from build123d import *

# Parameters (mm, degrees)
SKETCH1_R           = 2.5
SKETCH1_R_2         = 0.5
BOSS_EXTRUDE2_DEPTH = 4.572


with BuildPart() as part:
    # Sketch1 → Boss-Extrude2 (new body)
    with BuildSketch(Plane.XY):
        with BuildLine():
            Line((4.800174543, 7.530126516), (4.800174543, 44.360126516))
            ThreePointArc((4.800174543, 44.360126516), (4.056225767, 46.15617774), (2.260174543, 46.900126516))
            Line((2.260174543, 46.900126516), (-2.819825457, 46.900126516))
            ThreePointArc((-2.819825457, 46.900126516), (-4.615876681, 46.15617774), (-5.359825457, 44.360126516))
            Line((-5.359825457, 44.360126516), (-5.359825457, -5.169873484))
            Line((-5.359825457, -5.169873484), (-5.359825457, -47.079873484))
            ThreePointArc((-5.359825457, -47.079873484), (28.060725855, -35.300861478), (46.710174543, -5.169873484))
            Line((46.710174543, -5.169873484), (46.710174543, -2.629873484))
            Line((46.710174543, -2.629873484), (46.710174543, 2.450126516))
            ThreePointArc((46.710174543, 2.450126516), (45.966225767, 4.24617774), (44.170174543, 4.990126516))
            Line((44.170174543, 4.990126516), (7.340174543, 4.990126516))
            ThreePointArc((7.340174543, 4.990126516), (5.544123319, 5.734075291), (4.800174543, 7.530126516))
        make_face()
        Circle(SKETCH1_R, mode=Mode.SUBTRACT)
        with Locations((0, 11.43)):
            Circle(SKETCH1_R_2, mode=Mode.SUBTRACT)
        with Locations((11.43, 0)):
            Circle(SKETCH1_R_2, mode=Mode.SUBTRACT)
        with Locations((0, 13.97)):
            Circle(SKETCH1_R_2, mode=Mode.SUBTRACT)
        with Locations((13.97, 0)):
            Circle(SKETCH1_R_2, mode=Mode.SUBTRACT)
    extrude(amount=BOSS_EXTRUDE2_DEPTH)


solid = part.part
Can you work these out from the model? Positions are in its coordinate system, mm. A direction names the side the tool comes from. Round coordinates to 2 decimals unless told otherwise and drop trailing zeros. Write each loop counter-clockwise with the first axis right and the second up, starting at its lowest first coordinate (ties: lowest second). Pieces come first, ordered by that corner, then holes. Notation, with made-up numbers: M 47,42 L 63,42 A12 ccw 63,65 Z; hole C 34.25,56 d6. An arc over 180 degrees is marked long. Use a Markdown table: item, result.
Item 1: If I drill on line 1 along Y through (x, z) = (0, 2.15); line 2 along Y through (x, z) = (2, 0.2); line 3 along Y through (x, z) = (13.97, 1.65), over which ranges is the centre line in solid material (lowest first)? Write a range as [from, to].
Found:
| item | result |
|---|---|
| line 1 | y = [-46.81, -2.5], [2.5, 10.93], [11.93, 13.47], [14.47, 46.9] |
| line 2 | y = [-46.57, -1.5], [1.5, 46.9] |
| line 3 | y = [-43.45, -0.5], [0.5, 4.99] |
Item 2: Which directions (+Z, -Z, +X, -X, +Y, -Y) give clear straight access to the entire face, cutting with the end or side of a thin tool? Please do faces 5 (the face through (27.665, -35.616, 2.254)), 6 (the face through (4.8, 26, 2)).
Found:
| item | result |
|---|---|
| face 5 | +Z, -Z, +X, -Y |
| face 6 | +Z, -Z, +X, +Y |
Item 3: I want a section at B-B (y = 38). List the corners of the cut face in (x, z) for me.
Found:
| item | result |
|---|---|
| outline | M -5.36,0 L 4.8,0 L 4.8,4.57 L -5.36,4.57 Z |
Item 4: I want a section at A-A (z = 2.9). List the corners of the cut face in (x, y) for me.
Found:
| item | result |
|---|---|
| outline | M -5.36,-47.08 A53.3 ccw 46.71,-5.17 L 46.71,2.45 A2.54 ccw 44.17,4.99 L 7.34,4.99 A2.54 cw 4.8,7.53 L 4.8,44.36 A2.54 ccw 2.26,46.9 L -2.82,46.9 A2.54 ccw -5.36,44.36 Z; hole C 0,0 d5; hole C 0,11.43 d1; hole C 0,13.97 d1; hole C 11.43,0 d1; hole C 13.97,0 d1 |
Item 5: We'd pull the mould along X, two halves only. Please class faces 1 (the face through (26, 4.99, 2)), 2 (the face through (-0.54, -2.44, 2.25)), 3 (the face through (46.71, -1, 2)), 4 (the face through (-5.36, -1, 2)): released by +X, released by -X, zero draft, split by the parting line, or undercut.
Found:
| item | result |
|---|---|
| face 1 | zero draft |
| face 2 | undercut |
| face 3 | released by +X |
| face 4 | released by -X |
Item 6: I want a section at C-C (x = 10). List the corners of the cut face in (y, z) for me, and give its area (3 significant figures).
Found:
| item | result |
|---|---|
| outline | M -44.82,0 L 4.99,0 L 4.99,4.57 L -44.82,4.57 Z |
| area | 228 mm2 |
Item 7: For pin 1 Ø4.5 at (x, y) = (0, 0) entering from -Z; pin 2 Ø1 at (x, z) = (2.5, 1) entering from -Y, each with a flat end and sliding along its axis, tell me the tip position at first contact or that it passes through.
Found:
| item | result |
|---|---|
| pin 1 | passes through |
| pin 2 | stops at y = -46.57 |
